from build123d import *

# Parameters (mm, degrees)
F0_R     = 10.5
F1_DEPTH = 1
F2_R     = 6.5
F3_DEPTH = 1
F5_DEPTH = 3
F6_T     = -0.8
F7_SIZE  = 0.5


with BuildPart() as f1:
    # F0 (on Top) → F1 (new body)
    with BuildSketch(Plane.XY):
        Circle(F0_R)
    extrude(amount=F1_DEPTH)

    # F2 (on face) → F3 (join)
    with BuildSketch(Plane.XY.offset(1)):
        Circle(F2_R)
    extrude(amount=F3_DEPTH)

    # F4 (on face) → F5 (join)
    with BuildSketch(Plane.XY.offset(2)):
        Polygon((3.5507041555, 2.05), (0, 4.1), (-3.5507041555, 2.05), (-3.5507041555, -2.05), (0, -4.1), (3.5507041555, -2.05), align=None)
    extrude(amount=F5_DEPTH)

    # F6
    f6_openings = [f1.faces().sort_by_distance(p)[0] for p in [
        (0, 0, 5),
    ]]
    offset(amount=F6_T, openings=f6_openings, kind=Kind.INTERSECTION)

    # F7
    f7_edges = [f1.edges().sort_by_distance(p)[0] for p in [
        (-10.5, 0, 0),
    ]]
    chamfer(f7_edges, length=F7_SIZE)


solid = f1.part
CAD build for the part. Positions are in the model's coordinates, mm. A direction names the side the tool comes from. Give positions to 0.01 mm unless a question says otherwise; leave off trailing zeros. Write each loop counter-clockwise with the first axis right and the second up, starting at its lowest first coordinate (ties: lowest second). Pieces come first, ordered by that corner, then holes. Notation, with made-up numbers: (-36, 4) - (-21, 4) arc R14 cw to (-21, 11) - close; hole circle Ø3 at (84.25, 84.5). An arc over 180 degrees is marked (long way). Put each result on its own line as item: value.
(1) Wall check: L1, parallel to X at y = 0, z = 4.45; L2, parallel to Y at x = 0, z = 1.05; L3, parallel to Z at x = 4.5, y = 1.25. Give the ranges that are in metal, low to high.
Working result:
L1: -3.55 to -2.75, 2.75 to 3.55
L2: -6.5 to -5.7, 5.7 to 6.5
L3: 0 to 0.8, 1.2 to 2
(2) Tool access for faces 4 (the flat face through (-3.551, 0, 3)), 5 (the flat face through (1.36, -2.39, 3.07)), 6 (the flat face through (-1.8, -3.06, 3.48)), 7 (the flat face through (-1.75, 3.09, 3.48)), 8 (the cylindrical face through (10, 3.2, 0.7)): list every direction of +Z, -Z, +X, -X, +Y, -Y with a clear straight run to the whole face (end or side of a thin tool).
Working result:
face 4: +Z, -X, +Y, -Y
face 5: +Z
face 6: +Z, -X, -Y
face 7: +Z, -X, +Y
face 8: +Z, -Z
(3) Drop flat-ended pins along their axis: pin 1 Ø2.5 at (y, z) = (0, 2.5) entering from +X; pin 2 Ø2 at (x, y) = (3.5, 4.5) entering from +Z; pin 3 Ø1 at (y, z) = (4.5, 1) entering from -X. Give the stop position or say it passes through.
Working result:
pin 1: x = 6.5
pin 2: z = 2
pin 3: x = -9.71
(4) Saw through at B-B (y = 0). List the corners of the cut face in (x, z).
Working result:
outline: (-10.5, 0.5) - (-10, 0) - (10, 0) - (10.5, 0.5) - (10.5, 1) - (6.5, 1) - (6.5, 2) - (3.55, 2) - (3.55, 5) - (2.75, 5) - (2.75, 1.2) - (5.7, 1.2) - (5.7, 0.8) - (-5.7, 0.8) - (-5.7, 1.2) - (-2.75, 1.2) - (-2.75, 5) - (-3.55, 5) - (-3.55, 2) - (-6.5, 2) - (-6.5, 1) - (-10.5, 1) - close
(5) Saw through at A-A (z = 3.55). List the corners of the cut face in (x, y).
Working result:
outline: (-3.55, -2.05) - (0, -4.1) - (3.55, -2.05) - (3.55, 2.05) - (0, 4.1) - (-3.55, 2.05) - close; hole (-2.75, -1.59) - (0, -3.18) - (2.75, -1.59) - (2.75, 1.59) - (0, 3.18) - (-2.75, 1.59) - close
(6) Pull direction Z, two halves, no side cores. Call faces 1 (the flat face through (0, 0, 0.8)), 2 (the flat face through (1.8, 3.06, 3.48)), 3 (the flat face through (3, -3, 2)): released by +Z, released by -Z, zero draft, split by the parting line, or undercut.
Working result:
face 1: undercut
face 2: zero draft
face 3: released by +Z
